```python
from build123d import *
from build123d.topology import SkipClean

# Parameters (mm, degrees)
ESQUISSE1_R                                = 30
BOSS_EXTRU_1_DEPTH                         = 15
ESQUISSE2_R                                = 12.5
BOSS_EXTRU_2_DEPTH                         = 124
ESQUISSE4_2_W                              = 230
ESQUISSE4_2_H                              = 40
ENL_V_MAT_EXTRU_1_DEPTH                    = 5
CHAMBRAGE_POUR_VIS_T_TE_HEXAGONALE_2_COUNT = 2
CHAMBRAGE_POUR_VIS_T_TE_HEXAGONALE_2_PITCH = 41
ESQUISSE17_R                               = 6
BOSS_EXTRU_4_DEPTH                         = 83.38
ESQUISSE18_W                               = 10.356322474
ESQUISSE18_H                               = 3
ENL_V_MAT_EXTRU_2_DEPTH                    = 3
ESQUISSE19_W                               = 7.933443835
ESQUISSE19_H                               = 21.9317122
ENL_V_MAT_EXTRU_3_DEPTH                    = 50
BOSS_EXTRU_6_START                         = -10
ESQUISSE21_R                               = 12.5
BOSS_EXTRU_6_DEPTH                         = 10
D_GAGEMENT_M41_D                           = 4.5
D_GAGEMENT_M41_DEPTH                       = 3
D_GAGEMENT_M41_TIP                         = 1.299038106
ESQUISSE26_R                               = 17.5
BOSS_EXTRU_8_DEPTH                         = 52
ENL_V_START                                = -32
ESQUISSE27_R                               = 17.5
ENL_V_MAT_EXTRU_5_DEPTH                    = 32
ENL_V_START_2                              = -15
ESQUISSE28_R                               = 30
ENL_V_MAT_EXTRU_6_DEPTH                    = 15
BOSS_EXTRU_9_START                         = 10
BOSS_EXTRU_9_DEPTH                         = 10
D_GAGEMENT_M61_D                           = 6.6
D_GAGEMENT_M61_DEPTH                       = 4
D_GAGEMENT_M61_TIP                         = 1.905255888


with BuildPart() as part:
    # Esquisse1 → Boss.-Extru.1 (new body)
    with BuildSketch(Plane.XY):
        Circle(ESQUISSE1_R)
    extrude(amount=BOSS_EXTRU_1_DEPTH)

    # Esquisse2 → Boss.-Extru.2 (add)
    with BuildSketch(Plane(origin=(0, 0, 0), x_dir=(-1, 0, 0), z_dir=(0, 0, -1))):
        with Locations(Location((0, 0, 0), (0, 0, 180))):
            Circle(ESQUISSE2_R)
    extrude(amount=BOSS_EXTRU_2_DEPTH)

    # Esquisse4_2 → Enl_v. mat.-Extru.1 (cut)
    with BuildSketch(Plane.XY.offset(15)):
        Rectangle(ESQUISSE4_2_W, ESQUISSE4_2_H)
    extrude(amount=-ENL_V_MAT_EXTRU_1_DEPTH, mode=Mode.SUBTRACT)

    # Esquisse14 → Chambrage pour vis _ t_te hexagonale M51 (revolve, cut)
    with BuildSketch(Plane.YZ.offset(-20.5)):
        Polygon((0, 0), (0, 15), (2.75, 15), (2.75, 3.605), (2.775, 3.58), (6.12, 3.58), (6.12, 0), align=None)
    chambrage_pour_vis_t_te_hexagonale_m51 = revolve(axis=Axis((-20.5, 0, -6.35), (0, 0, 1)), mode=Mode.SUBTRACT)

    # Chambrage pour vis _ t_te hexagonale 2: Chambrage pour vis _ t_te hexagonale M51 ×2
    with Locations(*[(i * CHAMBRAGE_POUR_VIS_T_TE_HEXAGONALE_2_PITCH, 0, 0) for i in range(1, CHAMBRAGE_POUR_VIS_T_TE_HEXAGONALE_2_COUNT)]):
        add(chambrage_pour_vis_t_te_hexagonale_m51, mode=Mode.SUBTRACT)

    # Esquisse17 → Boss.-Extru.4 (add)
    with BuildSketch(Plane(origin=(0, 0, -124), x_dir=(-1, 0, 0), z_dir=(0, 0, -1))):
        Circle(ESQUISSE17_R)
    extrude(amount=BOSS_EXTRU_4_DEPTH)

    # Esquisse18 → Enl_v. mat.-Extru.2 (cut)
    with BuildSketch(Plane(origin=(0, 0, -207.38), x_dir=(-1, 0, 0), z_dir=(0, 0, -1))):
        with Locations((1.787207702, 0)):
            Rectangle(ESQUISSE18_W, ESQUISSE18_H)
    extrude(amount=-ENL_V_MAT_EXTRU_2_DEPTH, mode=Mode.SUBTRACT)

    # Esquisse19 → Enl_v. mat.-Extru.3 (cut)
    with BuildSketch(Plane(origin=(0, 0, -124), x_dir=(-1, 0, 0), z_dir=(0, 0, -1))):
        with Locations((9.966721917, 0)):
            Rectangle(ESQUISSE19_W, ESQUISSE19_H)
    extrude(amount=-ENL_V_MAT_EXTRU_3_DEPTH, mode=Mode.SUBTRACT)

    # Esquisse21 → Boss.-Extru.6 (add)
    with BuildSketch(Plane(origin=(0, 0, -124), x_dir=(-1, 0, 0), z_dir=(0, 0, -1)).offset(BOSS_EXTRU_6_START)):
        with Locations(Location((0, 0, 0), (0, 0, 180))):
            Circle(ESQUISSE21_R)
    extrude(amount=BOSS_EXTRU_6_DEPTH)

    # D_gagement M41
    with Locations(Plane.ZY.offset(6)):
        with Locations((-82.1, 5.85067254), (-93.1, -2.14932746), (-93.1, 5.85067254), (-104.1, 5.85067254)):
            Hole(D_GAGEMENT_M41_D / 2, depth=D_GAGEMENT_M41_DEPTH)
            with Locations((0, 0, -(D_GAGEMENT_M41_DEPTH + D_GAGEMENT_M41_TIP / 2))):  # 120° drill point
                Cone(0, D_GAGEMENT_M41_D / 2, D_GAGEMENT_M41_TIP, mode=Mode.SUBTRACT)

    # Esquisse26 → Boss.-Extru.8 (add)
    with BuildSketch(Plane(origin=(0, 0, -74), x_dir=(-1, 0, 0), z_dir=(0, 0, -1))):
        Circle(ESQUISSE26_R)
    extrude(amount=-BOSS_EXTRU_8_DEPTH)

    # Esquisse27 → Enl_v. mat.-Extru.5 (cut)
    with SkipClean():  # the faces are left unmerged after this step: merging them gives an invalid solid
        with BuildSketch(Plane(origin=(0, 0, -74), x_dir=(-1, 0, 0), z_dir=(0, 0, -1)).offset(ENL_V_START)):
            Circle(ESQUISSE27_R)
            with BuildLine():
                ThreePointArc((6, 10.9658561), (10.752906584, 6.373774392), (12.5, 0))
                ThreePointArc((12.5, 0), (10.752906584, -6.373774392), (6, -10.9658561))
                ThreePointArc((6, -10.9658561), (-12.5, 0), (6, 10.9658561))
            make_face(mode=Mode.SUBTRACT)
        extrude(amount=ENL_V_MAT_EXTRU_5_DEPTH, mode=Mode.SUBTRACT)

    # Esquisse28 → Enl_v. mat.-Extru.6 (cut)
    with SkipClean():  # the faces are left unmerged after this step: merging them gives an invalid solid
        with BuildSketch(Plane.XY.offset(15).offset(ENL_V_START_2)):
            Circle(ESQUISSE28_R)
        extrude(amount=ENL_V_MAT_EXTRU_6_DEPTH, mode=Mode.SUBTRACT)

    # Esquisse29 → Boss.-Extru.9 (add)
    with SkipClean():  # the faces are left unmerged after this step: merging them gives an invalid solid
        with BuildSketch(Plane.XY.offset(BOSS_EXTRU_9_START)):
            with BuildLine():
                Line((-4, -11.842719282), (-4, -8.5))
                Line((-4, -8.5), (4, -8.5))
                Line((4, -8.5), (4, -11.842719282))
                ThreePointArc((4, -11.842719282), (10.155048006, -7.288689869), (12.5, 0))
                ThreePointArc((12.5, 0), (-7.288689869, 10.155048006), (-4, -11.842719282))
            make_face()
        extrude(amount=-BOSS_EXTRU_9_DEPTH)

    # D_gagement M61
    with Locations(Plane.XY.offset(10)):
        with Locations((0, 0)):
            Hole(D_GAGEMENT_M61_D / 2, depth=D_GAGEMENT_M61_DEPTH)
            with Locations((0, 0, -(D_GAGEMENT_M61_DEPTH + D_GAGEMENT_M61_TIP / 2))):  # 120° drill point
                Cone(0, D_GAGEMENT_M61_D / 2, D_GAGEMENT_M61_TIP, mode=Mode.SUBTRACT)


solid = part.part
```
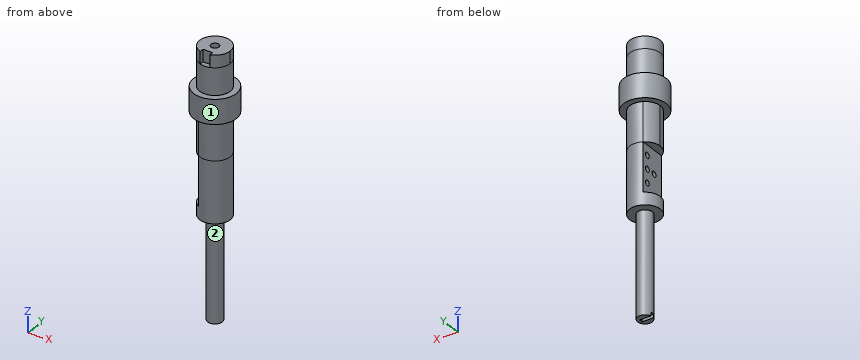
Work out the finished part from the listing and answer in its coordinate system (mm). Face numbers are marked on the shaded views. A direction names the side the tool comes from. Give positions to 0.01 mm unless a question says otherwise; leave off trailing zeros. Write each loop counter-clockwise with the first axis right and the second up, starting at its lowest first coordinate (ties: lowest second). Pieces come first, ordered by that corner, then holes.
(1) Flat-ended cylindrical pins translate along their axes: pin 1 Ø2.5 at (x, z) = (2, 6.5) entering from -Y; pin 2 Ø5 at (x, y) = (-8, -5.5) entering from -Z; pin 3 Ø3.5 at (y, z) = (5.85, -93.1) entering from -X. Find the tip coordinate at first contact, or state that the pin passes through.
Final values:
pin 1: stops at y = -8.5
pin 2: stops at z = -124
pin 3: stops at x = -2.71
(2) Which of the six approach directions +Z, -Z, +X, -X, +Y, -Y give full straight-line access (tool end or side, diameter ignored) to the marked faces 1 and 2?
Final values:
face 1: +Z, -Z
face 2: -Z
(3) The part is cut by section A-A on z = -24. Write down the section's boundary in (x, y), plus the area to 3 significant figures.
Final values:
outline: circle Ø35 at (0, 0)
area: 962 mm2
(4) Straight lines are drawn through the part: line 1 (Y direction, x = -4.35, z = -93.1); line 2 (Y direction, x = -5.15, z = -93.1); line 3 (Z direction, x = 7.5, y = -0.5). For each, find the intervals that lie inside material, in ascending order.
Final values:
line 1: y = -11.72 to -4.4, 0.1 to 3.6, 8.1 to 11.72
line 2: y = -11.39 to -4.4, 0.1 to 3.6, 8.1 to 11.39
line 3: z = -124 to 10
(5) The part is cut by section B-B on z = -144. Write down the section's boundary in (x, y).
Final values:
outline: circle Ø12 at (0, 0)
